```python
from build123d import *

# Parameters (mm, degrees)
SKETCH1_R               = 38.1
BOSS_EXTRUDE1_DEPTH     = 4
SKETCH2_R               = 1.1
CUT_EXTRUDE1_DEPTH      = 55.029806589
CUT_EXTRUDE2_DEPTH      = 55.029806589
CUT_EXTRUDE2_DEPTH_BACK = 55.029806589
SKETCH3_R               = 1.9304
CUT_EXTRUDE3_DEPTH      = 55.029806589
CUT_EXTRUDE3_DEPTH_BACK = 55.029806589
CUT_EXTRUDE4_REACH      = 56.03
SKETCH5_R               = 3.175
CUT_EXTRUDE5_REACH      = 56.03


with BuildPart() as part:
    # Sketch1 → Boss-Extrude1 (new body)
    with BuildSketch(Plane.XY):
        Circle(SKETCH1_R)
    extrude(amount=BOSS_EXTRUDE1_DEPTH)

    # Sketch2 → Cut-Extrude1 (cut, through all)
    with BuildSketch(Plane.XY.offset(4)):
        with Locations((10, 10)):
            Circle(SKETCH2_R)
        with Locations((10, -10)):
            Circle(SKETCH2_R)
        with Locations((-10, -10)):
            Circle(SKETCH2_R)
        with Locations((-10, 10)):
            Circle(SKETCH2_R)
    extrude(amount=-CUT_EXTRUDE1_DEPTH, mode=Mode.SUBTRACT)

    # Sketch3 → Cut-Extrude2 (cut, two sides: drawn at the far end of the back side and taken through both)
    with BuildSketch(Plane.XY.offset(4).offset(-CUT_EXTRUDE2_DEPTH_BACK)):
        with Locations((0, -31.75)):
            Circle(SKETCH3_R)
        with Locations((-31.75, 0)):
            Circle(SKETCH3_R)
        with Locations((0, 31.75)):
            Circle(SKETCH3_R)
        with Locations((31.75, 0)):
            Circle(SKETCH3_R)
    extrude(amount=CUT_EXTRUDE2_DEPTH + CUT_EXTRUDE2_DEPTH_BACK, mode=Mode.SUBTRACT)

    # Sketch4 → Cut-Extrude3 (cut, two sides: drawn at the far end of the back side and taken through both)
    with BuildSketch(Plane.XY.offset(4).offset(-CUT_EXTRUDE3_DEPTH_BACK)):
        with BuildLine():
            Line((-19.05, -8.89), (-26.67, -8.89))
            ThreePointArc((-26.67, -8.89), (-27.568025612, -8.518025612), (-27.94, -7.62))
            Line((-27.94, -7.62), (-27.94, 7.62))
            ThreePointArc((-27.94, 7.62), (-27.568025612, 8.518025612), (-26.67, 8.89))
            Line((-26.67, 8.89), (-19.05, 8.89))
            ThreePointArc((-19.05, 8.89), (-18.151974388, 8.518025612), (-17.78, 7.62))
            Line((-17.78, 7.62), (-17.78, -7.62))
            ThreePointArc((-17.78, -7.62), (-18.151974388, -8.518025612), (-19.05, -8.89))
        make_face()
        with BuildLine():
            Line((19.05, 8.89), (26.67, 8.89))
            ThreePointArc((26.67, 8.89), (27.568025612, 8.518025612), (27.94, 7.62))
            Line((27.94, 7.62), (27.94, -7.62))
            ThreePointArc((27.94, -7.62), (27.568025612, -8.518025612), (26.67, -8.89))
            Line((26.67, -8.89), (19.05, -8.89))
            ThreePointArc((19.05, -8.89), (18.151974388, -8.518025612), (17.78, -7.62))
            Line((17.78, -7.62), (17.78, 7.62))
            ThreePointArc((17.78, 7.62), (18.151974388, 8.518025612), (19.05, 8.89))
        make_face()
    extrude(amount=CUT_EXTRUDE3_DEPTH + CUT_EXTRUDE3_DEPTH_BACK, mode=Mode.SUBTRACT)

    # Sketch5 → Cut-Extrude4 (cut, up to next)
    with BuildSketch(Plane.XY.offset(4), mode=Mode.PRIVATE) as cut_extrude4_sk1:
        with Locations((0, 23.495)):
            Circle(SKETCH5_R)
    cut_extrude4_tool1 = extrude(cut_extrude4_sk1.sketch, amount=-CUT_EXTRUDE4_REACH, mode=Mode.PRIVATE) & part.part
    # Sketch5 → Cut-Extrude4 (cut, up to next)
    with BuildSketch(Plane.XY.offset(4), mode=Mode.PRIVATE) as cut_extrude4_sk2:
        with BuildLine():
            Line((-5.08, -27.305), (5.08, -27.305))
            ThreePointArc((5.08, -27.305), (5.978025612, -26.933025612), (6.35, -26.035))
            Line((6.35, -26.035), (6.35, -20.955))
            ThreePointArc((6.35, -20.955), (5.978025612, -20.056974388), (5.08, -19.685))
            Line((5.08, -19.685), (-5.08, -19.685))
            ThreePointArc((-5.08, -19.685), (-5.978025612, -20.056974388), (-6.35, -20.955))
            Line((-6.35, -20.955), (-6.35, -26.035))
            ThreePointArc((-6.35, -26.035), (-5.978025612, -26.933025612), (-5.08, -27.305))
        make_face()
    cut_extrude4_tool2 = extrude(cut_extrude4_sk2.sketch, amount=-CUT_EXTRUDE4_REACH, mode=Mode.PRIVATE) & part.part
    add(cut_extrude4_tool1.solids().sort_by_distance((0, 23.495, 4))[0], mode=Mode.SUBTRACT)
    add(cut_extrude4_tool2.solids().sort_by_distance((0, -23.495, 4))[0], mode=Mode.SUBTRACT)

    # Sketch6 → Cut-Extrude5 (cut, up to next)
    with BuildSketch(Plane.XY.offset(4), mode=Mode.PRIVATE) as cut_extrude5_sk1:
        Polygon((-18.415, 22.90700482), (-14.605, 22.90700482), (-14.605, 30.52700482), (-12.065, 30.52700482), (-12.065, 20.36700482), (-20.955, 20.36700482), (-20.955, 30.52700482), (-18.415, 30.52700482), align=None)
    cut_extrude5_tool1 = extrude(cut_extrude5_sk1.sketch, amount=-CUT_EXTRUDE5_REACH, mode=Mode.PRIVATE) & part.part
    # Sketch6 → Cut-Extrude5 (cut, up to next)
    with BuildSketch(Plane.XY.offset(4), mode=Mode.PRIVATE) as cut_extrude5_sk2:
        Polygon((22.90700482, 18.415), (22.90700482, 14.605), (30.52700482, 14.605), (30.52700482, 12.065), (20.36700482, 12.065), (20.36700482, 20.955), (30.52700482, 20.955), (30.52700482, 18.415), align=None)
    cut_extrude5_tool2 = extrude(cut_extrude5_sk2.sketch, amount=-CUT_EXTRUDE5_REACH, mode=Mode.PRIVATE) & part.part
    # Sketch6 → Cut-Extrude5 (cut, up to next)
    with BuildSketch(Plane.XY.offset(4), mode=Mode.PRIVATE) as cut_extrude5_sk3:
        Polygon((18.415, -22.90700482), (14.605, -22.90700482), (14.605, -30.52700482), (12.065, -30.52700482), (12.065, -20.36700482), (20.955, -20.36700482), (20.955, -30.52700482), (18.415, -30.52700482), align=None)
    cut_extrude5_tool3 = extrude(cut_extrude5_sk3.sketch, amount=-CUT_EXTRUDE5_REACH, mode=Mode.PRIVATE) & part.part
    # Sketch6 → Cut-Extrude5 (cut, up to next)
    with BuildSketch(Plane.XY.offset(4), mode=Mode.PRIVATE) as cut_extrude5_sk4:
        Polygon((-22.90700482, -18.415), (-22.90700482, -14.605), (-30.52700482, -14.605), (-30.52700482, -12.065), (-20.36700482, -12.065), (-20.36700482, -20.955), (-30.52700482, -20.955), (-30.52700482, -18.415), align=None)
    cut_extrude5_tool4 = extrude(cut_extrude5_sk4.sketch, amount=-CUT_EXTRUDE5_REACH, mode=Mode.PRIVATE) & part.part
    add(cut_extrude5_tool1.solids().sort_by_distance((-16.51, 22.772002, 4))[0], mode=Mode.SUBTRACT)
    add(cut_extrude5_tool2.solids().sort_by_distance((22.772002, 16.51, 4))[0], mode=Mode.SUBTRACT)
    add(cut_extrude5_tool3.solids().sort_by_distance((16.51, -22.772002, 4))[0], mode=Mode.SUBTRACT)
    add(cut_extrude5_tool4.solids().sort_by_distance((-22.772002, -16.51, 4))[0], mode=Mode.SUBTRACT)


solid = part.part
```
CAD build for the part. Positions are in the model's coordinates, mm. Round coordinates to 2 decimals unless told otherwise and drop trailing zeros. Order: outer loops, then holes, each group sorted by start corner. A loop starts at its lowest first (then second) coordinate and runs counter-clockwise, first axis right, second up. Notation, with made-up numbers: (58.25, 77.5) - (116.25, 77.5) arc R27 ccw to (116.25, 99.5) - close; hole circle Ø4 at (7, -2). An arc over 180 degrees is marked (long way). Use CSV: the item, a comma, the result in double quotes. Start each with the question number.
1) Wall check: L1, parallel to Y at x = 0, z = 1.7 (3 decimals); L2, parallel to X at y = -24.5, z = 2.35 (3 decimals); L3, parallel to Y at x = -22, z = 3.85 (3 decimals). Give the ranges that are in metal, low to high. Write a range as [from, to].
2) Saw through at A-A (x = 0). List the corners of the cut face in (y, z) (3 decimals), and give its area (3 significant figures).
3) Pin check, flat tips, straight feed: pin 1 Ø1.2 at (y, z) = (-22.5, 2) entering from -X; pin 2 Ø1.1 at (x, z) = (-16, 2) entering from -Y; pin 3 Ø1.8 at (x, y) = (-10, 10) entering from +Z; pin 4 Ø1.2 at (x, z) = (21, 2) entering from +Y. Stop position of each tip, or through.
4) Two-plate mould, pull along X, no slides. Class faces 1 (the flat face through (0, -19.685, 2)), 2 (the flat face through (22.907, 17, 2)), 3 (the cylindrical face through (-30.235, -23.183, 1.972)): pulls with the +X half, pulls with the -X half, needs draft (parallel to the pull), parting line crosses it, or undercut.
5) Saw through at D-D (x = 10). List the corners of the cut face in (y, z).
6) Saw through at B-B (y = 31.75). List the corners of the cut face in (x, z).
Values follow:
1,L1,"y = [-38.1, -33.68], [-29.82, -27.305], [-19.685, 20.32], [26.67, 29.82], [33.68, 38.1]"
1,L2,"x = [-29.178, -6.35], [6.35, 12.065], [14.605, 18.415], [20.955, 29.178]"
1,L3,"y = [-31.106, -20.955], [-12.065, -8.89], [8.89, 31.106]"
2,outline,"(-38.1, 0) - (-33.68, 0) - (-33.68, 4) - (-38.1, 4) - close; (-29.82, 0) - (-27.305, 0) - (-27.305, 4) - (-29.82, 4) - close; (-19.685, 0) - (20.32, 0) - (20.32, 4) - (-19.685, 4) - close; (26.67, 0) - (29.82, 0) - (29.82, 4) - (26.67, 4) - close; (33.68, 0) - (38.1, 0) - (38.1, 4) - (33.68, 4) - close"
2,area,"218 mm2"
3,pin 1,"stops at x = -31.18"
3,pin 2,"stops at y = -34.83"
3,pin 3,"passes through"
3,pin 4,"stops at y = 32.18"
4,face 1,"undercut"
4,face 2,"undercut"
4,face 3,"parting line crosses it"
5,outline,"(-36.76, 0) - (-11.1, 0) - (-11.1, 4) - (-36.76, 4) - close; (-8.9, 0) - (8.9, 0) - (8.9, 4) - (-8.9, 4) - close; (11.1, 0) - (36.76, 0) - (36.76, 4) - (11.1, 4) - close"
6,outline,"(-21.06, 0) - (-1.93, 0) - (-1.93, 4) - (-21.06, 4) - close; (1.93, 0) - (21.06, 0) - (21.06, 4) - (1.93, 4) - close"
